```python
from build123d import *

# Parameters (mm, degrees)
M3_TAPPED_HOLE1_D     = 2.5
M3_TAPPED_HOLE1_DEPTH = 7.5
M3_TAPPED_HOLE1_TIP   = 0.751075774
SKETCH4_OUTSIDE_W     = 111.87
SKETCH4_OUTSIDE_H     = 111.87
SKETCH4_OUTSIDE_W_2   = 40
SKETCH4_OUTSIDE_H_2   = 58.988764044
EXTRUDE1_DEPTH        = 30
M6_TAPPED_HOLE1_D     = 5


with BuildPart() as part:
    # Sketch1 → Revolve1 (revolve)
    with BuildSketch(Plane.XY, mode=Mode.PRIVATE) as revolve1_sk:
        Polygon((19, 66.959459459), (39, 66.959459459), (39, 56.959459459), (24, 56.959459459), (24, 36.959459459), (22, 36.959459459), (22, -48.040540541), (12.5, -48.040540541), (12.5, -41.040540541), (10.5, -41.040540541), (10.5, -34.040540541), (8.5, -34.040540541), (8.5, -14.040540541), (19, -14.040540541), align=None)
    revolve(revolve1_sk.sketch.rotate(Axis((0, 66.959459459, 0), (0, -1, 0)), 90), axis=Axis((0, 66.959459459, 0), (0, -1, 0)))

    # M3 Tapped Hole1
    with Locations(Plane(origin=(-11, -48.040540541, 11), x_dir=(0, 0, -1), z_dir=(0, -1, 0))):
        with Locations((0, 0), (0, 22), (22, 0), (22, 22)):
            Hole(M3_TAPPED_HOLE1_D / 2, depth=M3_TAPPED_HOLE1_DEPTH)
            with Locations((0, 0, -(M3_TAPPED_HOLE1_DEPTH + M3_TAPPED_HOLE1_TIP / 2))):  # 118° drill point
                Cone(0, M3_TAPPED_HOLE1_D / 2, M3_TAPPED_HOLE1_TIP, mode=Mode.SUBTRACT)

    # Sketch4 outside → Extrude1 (cut)
    with BuildSketch(Plane.XZ.offset(48.040540541)):
        Rectangle(SKETCH4_OUTSIDE_W, SKETCH4_OUTSIDE_H)
        Rectangle(SKETCH4_OUTSIDE_W_2, SKETCH4_OUTSIDE_H_2, mode=Mode.SUBTRACT)
    extrude(amount=-EXTRUDE1_DEPTH, mode=Mode.SUBTRACT)

    # M6 Tapped Hole1 (through all)
    with Locations(Plane(origin=(-20, -23.040540541, 0), x_dir=(0, 0, -1), z_dir=(-1, 0, 0))):
        with Locations((0, 0), (0, 20)):
            Hole(M6_TAPPED_HOLE1_D / 2)


solid = part.part
```
Work out the finished part from the listing and answer in its coordinate system (mm). A direction names the side the tool comes from. Give positions to 0.01 mm unless a question says otherwise; leave off trailing zeros. Order: outer loops, then holes, each group sorted by start corner. A loop starts at its lowest first (then second) coordinate and runs counter-clockwise, first axis right, second up. Notation, with made-up numbers: (72, 17) - (107, 17) arc R8 cw to (107, 23) - close; hole circle Ø2 at (57.25, -17). An arc over 180 degrees is marked (long way). One line per item, written item: value. Start each with the question number.
1. For a pull along Z with two mould halves and no side action, classify faces 1 (the face through (-3.2, -37.5, 10)), 2 (the face through (16.33, -40.6, -0.54)), 3 (the face through (-9, 66.959, -17)), 4 (the face through (-38.668, 61.889, -5.077)) as released by +Z, released by -Z, zero draft, split by the parting line, or undercut.
2. Which of the six approach directions +Z, -Z, +X, -X, +Y, -Y give full straight-line access (tool end or side, diameter ignored) to faces 5 (the face through (4, -14.041, -8)), 6 (the face through (0, -41.041, -11)), 7 (the face through (-2.55, -23.9, 8.11)), 8 (the face through (-20, -33, 0))?
3. Section B-B, the plane y = 40.5 is taken. Write down the section's boundary in (x, z), then the cut area to 3 significant figures.
4. Section A-A, the plane x = 0 is taken. Write down the section's boundary in (y, z).
5. Consider line 1 (Y direction, x = -16.25, z = 0); line 2 (X direction, y = -43.75, z = 11); line 3 (Z direction, x = 0.5, y = 52). Determine where each line is inside the solid, lowest interval first.
6. Section C-C, the plane z = 0 is taken. Count the separate pieces of the cut face and the enclosed holes in it, then the cut area to 3 significant figures.
7. Section D-D, the plane z = 17.5 is taken. Write down the section's boundary in (x, y).
8. Each of these flat-tipped pins is pushed along its axis until it touches: pin 1 Ø3 at (x, y) = (21, 5) entering from +Z; pin 2 Ø23 at (x, z) = (0.5, 3.5) entering from -Y; pin 3 Ø8 at (x, y) = (-0.5, 45) entering from +Z; pin 4 Ø3 at (x, z) = (-20.5, 12) entering from -Y. Where does it stop, or does it pass through?
Filled sheet:
1. face 1: undercut
1. face 2: undercut
1. face 3: zero draft
1. face 4: split by the parting line
2. face 5: +Y
2. face 6: -Y
2. face 7: +Y, -Y
2. face 8: +Z, -Z, -X, -Y
3. outline: circle Ø48 at (0, 0); hole circle Ø38 at (0, 0)
3. area: 675 mm²
4. outline: (-48.04, -22) - (36.96, -22) - (36.96, -24) - (56.96, -24) - (56.96, -39) - (66.96, -39) - (66.96, -19) - (-14.04, -19) - (-14.04, -8.5) - (-34.04, -8.5) - (-34.04, -10.5) - (-41.04, -10.5) - (-41.04, -12.5) - (-48.04, -12.5) - close; (-48.04, 12.5) - (-41.04, 12.5) - (-41.04, 10.5) - (-34.04, 10.5) - (-34.04, 8.5) - (-14.04, 8.5) - (-14.04, 19) - (66.96, 19) - (66.96, 39) - (56.96, 39) - (56.96, 24) - (36.96, 24) - (36.96, 22) - (-48.04, 22) - close
5. line 1: -48.04 to -45.54, -40.54 to -25.54, -20.54 to -14.04
5. line 2: -19.05 to -12.25, -9.75 to -5.94, 5.94 to 9.75, 12.25 to 19.05
5. line 3: -23.99 to -18.99, 18.99 to 23.99
6. separate pieces: 6
6. enclosed holes: 0
6. area: 1,430 mm²
7. outline: (-34.85, 56.96) - (-16.42, 56.96) - (-16.42, 36.96) - (-13.33, 36.96) - (-13.33, -48.04) - (13.33, -48.04) - (13.33, 36.96) - (16.42, 36.96) - (16.42, 56.96) - (34.85, 56.96) - (34.85, 66.96) - (7.4, 66.96) - (7.4, -14.04) - (-7.4, -14.04) - (-7.4, 66.96) - (-34.85, 66.96) - close
8. pin 1: z = 10.19
8. pin 2: y = -48.04
8. pin 3: z = 24
8. pin 4: y = 36.96
